from build123d import *

# Parameters (mm, degrees)
CROQUIS1_W              = 15
CROQUIS1_H              = 5
SALIENTE_EXTRUIR1_DEPTH = 5
CROQUIS2_R              = 1.7
CORTAR_EXTRUIR1_DEPTH   = 6
CROQUIS3_R              = 1.25
CORTAR_EXTRUIR2_DEPTH   = 6


with BuildPart() as part:
    # Croquis1 → Saliente-Extruir1 (new body)
    with BuildSketch(Plane(origin=(0, 0, 0), x_dir=(1, 0, 0), z_dir=(0, 1, 0))):
        Rectangle(CROQUIS1_W, CROQUIS1_H)
    extrude(amount=SALIENTE_EXTRUIR1_DEPTH)

    # Croquis2 → Cortar-Extruir1 (cut, through all)
    with BuildSketch(Plane(origin=(0, 5, 0), x_dir=(1, 0, 0), z_dir=(0, 1, 0))):
        with Locations((-5, 0)):
            Circle(CROQUIS2_R)
        with Locations((5, 0)):
            Circle(CROQUIS2_R)
    extrude(amount=-CORTAR_EXTRUIR1_DEPTH, mode=Mode.SUBTRACT)

    # Croquis3 → Cortar-Extruir2 (cut, through all)
    with BuildSketch(Plane.XY.offset(2.5)):
        with Locations((0, 2.5)):
            Circle(CROQUIS3_R)
    extrude(amount=-CORTAR_EXTRUIR2_DEPTH, mode=Mode.SUBTRACT)


solid = part.part
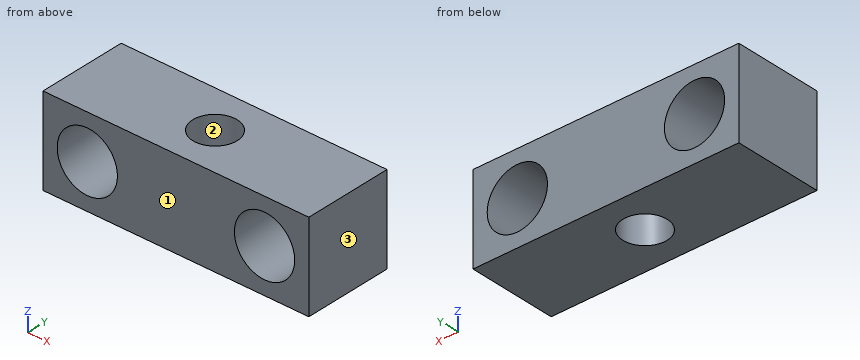
The listing builds one solid part. Answer for the finished solid, in the listing's coordinates (mm). Face numbers are marked on the shaded views. Coordinates: 2 decimals unless noted, no trailing zeros. Write each loop counter-clockwise with the first axis right and the second up, starting at its lowest first coordinate (ties: lowest second). Pieces come first, ordered by that corner, then holes. Notation, with made-up numbers: M -2,50 L 14,50 A14 ccw 14,67 Z; hole C 41,17 d8. An arc over 180 degrees is marked long. Put each result on its own line as item: value. Start each with the question number.
1. For a pull along Y with two mould halves and no side action, classify the marked faces 1, 2 and 3 as pulls with the +Y half, pulls with the -Y half, needs draft (parallel to the pull), parting line crosses it, or undercut.
2. A flat-ended cylindrical pin translates along its axis: P1, Ø2.5, axis at x = 5, z = 0, coming from the +Y side. Find the tip coordinate at first contact, or state that the pin passes through.
3. A cutting plane is placed at A-A on z = 0. Write down the section's boundary in (x, y), then the cut area to 3 significant figures.
4. A cutting plane is placed at C-C on x = -3.5. Write down the section's boundary in (y, z).
5. A cutting plane is placed at B-B on y = 2.5. Write down the section's boundary in (x, z), then the cut area to 3 significant figures.
6. Consider line 1 (X direction, y = 2.55, z = 1.9); line 2 (X direction, y = 4.65, z = -0.95); line 3 (X direction, y = 4.6, z = 1.1). Determine where each line is inside the solid, lowest interval first. Write a range as from..to.
7. A cutting plane is placed at D-D on z = 2.05. Write down the section's boundary in (x, y), then the cut area to 3 significant figures.
Resolved:
1. face 1: pulls with the -Y half
1. face 2: undercut
1. face 3: needs draft
2. P1: passes through
3. outline: M -7.5,0 L -6.7,0 L -6.7,5 L -7.5,5 Z; M -3.3,0 L 3.3,0 L 3.3,5 L -3.3,5 Z; M 6.7,0 L 7.5,0 L 7.5,5 L 6.7,5 Z; hole C 0,2.5 d2.5
3. area: 36.1 mm2
4. outline: M 0,-2.5 L 5,-2.5 L 5,-0.8 L 0,-0.8 Z; M 0,0.8 L 5,0.8 L 5,2.5 L 0,2.5 Z
5. outline: M -7.5,-2.5 L -1.25,-2.5 L -1.25,2.5 L -7.5,2.5 Z; M 1.25,-2.5 L 7.5,-2.5 L 7.5,2.5 L 1.25,2.5 Z; hole C -5,0 d3.4; hole C 5,0 d3.4
5. area: 44.3 mm2
6. line 1: x = -7.5..-1.25, 1.25..7.5
6. line 2: x = -7.5..-6.41, -3.59..3.59, 6.41..7.5
6. line 3: x = -7.5..-6.3, -3.7..3.7, 6.3..7.5
7. outline: M -7.5,0 L 7.5,0 L 7.5,5 L -7.5,5 Z; hole C 0,2.5 d2.5
7. area: 70.1 mm2
